The model under review builds one solid part; all positions refer to its coordinate system, in mm. Face numbers are marked on the shaded views. Round coordinates to 2 decimals unless told otherwise and drop trailing zeros. Loops run counter-clockwise (first coordinate to the right, second up) from the corner with the lowest first, then second, coordinate; pieces in that order, holes last. Notation, with made-up numbers: (-0.5, 15) - (6.5, 15) arc R21 ccw to (6.5, 40) - close; hole circle Ø1 at (35.25, -30.5). An arc over 180 degrees is marked (long way). Answer as CSV lines item,"result".
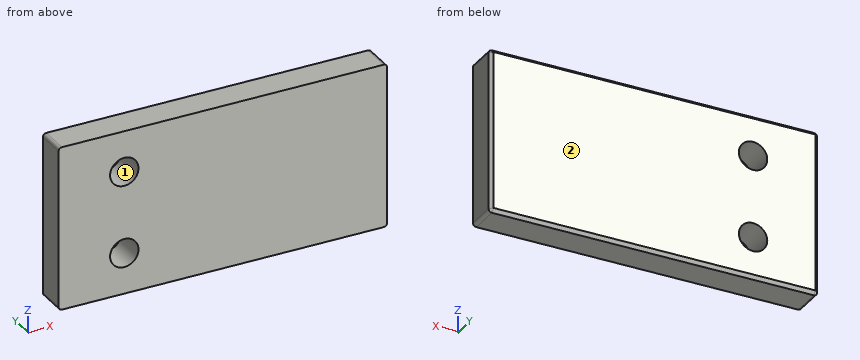
from build123d import *

# Parameters (mm, degrees)
SKETCH_1_W          = 100
SKETCH_1_H          = 50
EXTRUDE_1_DEPTH     = 10
FILLET_1_R          = 1
CHAMFER_2_SIZE      = 1
HOLE_WIZARD_1_D     = 8.647
HOLE_WIZARD_1_DEPTH = 26.2
HOLE_WIZARD_1_TIP   = 2.597820886


with BuildPart() as part:
    # 草圖1 → 擠出1 (new body)
    with BuildSketch(Plane(origin=(0, 0, 0), x_dir=(-1, 0, 0), z_dir=(0, 1, 0))):
        Rectangle(SKETCH_1_W, SKETCH_1_H)
    extrude(amount=EXTRUDE_1_DEPTH)

    # 圓角1
    fillet_1_edges = [part.edges().sort_by_distance(p)[0] for p in [
        (-50, 5, -25),
        (50, 5, -25),
        (50, 5, 25),
        (-50, 5, 25),
    ]]
    fillet(fillet_1_edges, radius=FILLET_1_R)

    # 倒角2
    chamfer_2_edges = [part.edges().sort_by_distance(p)[0] for p in [
        (0, 10, 25),
        (-50, 10, 0),
        (50, 10, 0),
        (0, 10, -25),
        (49.707106781, 10, 24.707106781),
        (49.707106781, 10, -24.707106781),
        (-49.707106781, 10, -24.707106781),
        (-49.707106781, 10, 24.707106781),
    ]]
    chamfer(chamfer_2_edges, length=CHAMFER_2_SIZE)

    # 孔1
    with Locations(Plane(origin=(0, 10, 0), x_dir=(1, 0, 0), z_dir=(0, 1, 0))):
        with Locations((-30, 12.5), (-30, -12.5)):
            Hole(HOLE_WIZARD_1_D / 2, depth=HOLE_WIZARD_1_DEPTH)
            with Locations((0, 0, -(HOLE_WIZARD_1_DEPTH + HOLE_WIZARD_1_TIP / 2))):  # 118° drill point
                Cone(0, HOLE_WIZARD_1_D / 2, HOLE_WIZARD_1_TIP, mode=Mode.SUBTRACT)


solid = part.part
1. Take a section at B-B (y = 3). State the section outline as (x, z) points, plus the area to 3 significant figures.
Numbers:
outline,"(-50, -24) arc R1 ccw to (-49, -25) - (49, -25) arc R1 ccw to (50, -24) - (50, 24) arc R1 ccw to (49, 25) - (-49, 25) arc R1 ccw to (-50, 24) - close; hole circle Ø8.65 at (-30, -12.5); hole circle Ø8.65 at (-30, 12.5)"
area,"4,880 mm²"
2. Take a section at C-C (x = -30). State the section outline as (y, z) points, plus the area to 3 significant figures.
Numbers:
outline,"(0, -25) - (9, -25) - (10, -24) - (10, -16.82) - (0, -16.82) - close; (0, -8.18) - (10, -8.18) - (10, 8.18) - (0, 8.18) - close; (0, 16.82) - (10, 16.82) - (10, 24) - (9, 25) - (0, 25) - close"
area,"326 mm²"
3. Draft analysis for pull direction X (two halves, no side actions). For the marked faces 1 and 2, state which applies: +X half, -X half, draft (parallel to the pull), parting line (faces both ways), or undercut.
Numbers:
face 1,"undercut"
face 2,"draft"
4. Wall thickness on probe 1 along Z at (x, y) = (-30, 7); probe 2 along Z at (x, y) = (-29, 6.5); probe 3 along X at (y, z) = (9.75, -16.5): over which ranges is each line inside the solid? List them lowest first.
Numbers:
probe 1,"z = -25 to -16.82, -8.18 to 8.18, 16.82 to 25"
probe 2,"z = -25 to -16.71, -8.29 to 8.29, 16.71 to 25"
probe 3,"x = -49.25 to -31.64, -28.36 to 49.25"
5. Clearance check with a flat-ended pin moving along its axis: pin 1 (12 mm diameter, centred on x = 26, z = 14, fed in from -Y). State where the tip first meets the part, or that it passes through.
Numbers:
pin 1,"stops at y = 0"
6. Take a section at A-A (z = -12.5). State the section outline as (x, y) points, plus the area to 3 significant figures.
Numbers:
outline,"(-50, 0) - (-34.32, 0) - (-34.32, 10) - (-49, 10) - (-50, 9) - close; (-25.68, 0) - (50, 0) - (50, 9) - (49, 10) - (-25.68, 10) - close"
area,"913 mm²"
